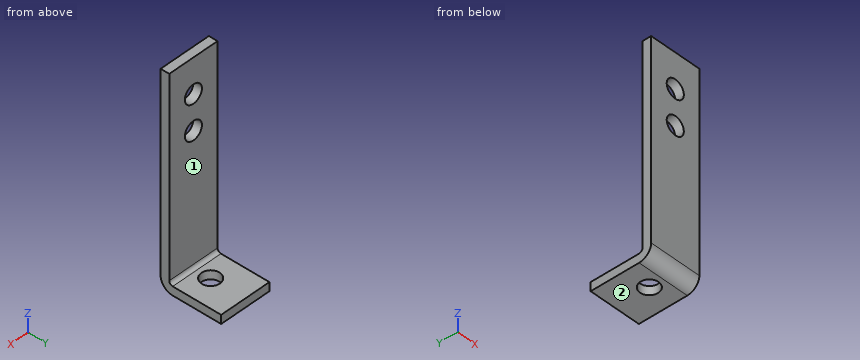
Autodesk Inventor part; units mm, degrees
ref_plane "YZ Plane" through (0, 0, 0) normal (1, 0, 0) x (0, 1, 0)
ref_plane "XZ Plane" through (0, 0, 0) normal (0, 1, 0) x (-1, 0, 0)
ref_plane "XY Plane" through (0, 0, 0) normal (0, 0, 1) x (1, 0, 0)
sketch "Sketch1" plane through (0, 0, 0) normal (0, 0, 1) x (1, 0, 0)
  line L0 (0, 0) -> (0, -22.225)
  line L1 (0, 0) -> (-19.05, 0)
  line L2 (-19.05, 0) -> (-19.05, -22.225)
  line L3 (-19.05, -22.225) -> (0, -22.225)
  dimension "d0" = 22.225
  dimension "d1" = 19.05
extrude "Plate1" add sketch "Sketch1" along normal blind 3.175
sketch "Sketch2" plane through (0, -19.05, 0) normal (0, -1, 0) x (1, 0, 0)
  line L0 (-19.05, 0) -> (0, 0)
  line L1 (0, 0) -> (0, 76.2)
  line L2 (0, 76.2) -> (-19.05, 76.2)
  line L3 (-19.05, 76.2) -> (-19.05, 0)
edge flange "Flange1" height 76.2 angle 90 thickness 3.175 bend radius 1.27 thickness toward (0, -1, 0) relief straight relief width 3.175 relief depth 1.5875 edges at (-9.525, -22.225, 3.175) wall of the first edge with corners at (-19.05, -19.05, 0) (0, -19.05, 0) (0, -19.05, 76.2) (-19.05, -19.05, 76.2)
bend "Bend1"
corner "Corner1"
sketch "Sketch3" plane through (0, 0, 3.175) normal (0, 0, 1) x (1, 0, 0)
  circle A0 centre (90.7515, -113.3098) radius 3.3782
  circle A1 centre (90.7515, -113.3098) radius 3.3782
  circle A2 centre (-9.525, -12.7) radius 3.3782
extrude "Cut1" cut sketch "Sketch3" against normal blind 3.175 contours A2
sketch "Sketch4" plane through (-19.05, -19.05, 76.2) normal (0, 1, 0) x (1, 0, 0)
  line L0 (0, 0) -> (19.05, 0)
  line L1 (19.05, 0) -> (19.05, 71.755)
  line L2 (9.525, 0) -> (9.525, 12.7)
  circle A0 centre (9.525, 12.7) radius 3.3782
  line L3 (9.525, 12.7) -> (9.525, 25.4)
  circle A1 centre (9.525, 25.4) radius 3.3782
  point P0 (19.05, 76.2)
  dimension "d15" = 12.7
  dimension "d16" = 6.7564
  dimension "d17" = 12.7
  dimension "d18" = 6.7564
extrude "Cut2" cut sketch "Sketch4" against normal blind 3.175
equation "\"d13\" = Thickness"
equation "\"d19\" = Thickness"
equation "\"d3\" = BendReliefWidth"
equation "\"d4\" = BendReliefDepth"
equation "\"d5\" = MinimumRemnant"
equation "\"d6\" = BendRadius"
equation "\"d10\" = CornerReliefSize"
equation "\"d11\" = GapSize"
equation "\"d12\" = JacobiRadiusSize"
equation "\"BendRadius\" = Thickness"
equation "\"BendReliefWidth\" = Thickness"
equation "\"BendReliefDepth\" = 0.5 * Thickness"
equation "\"CornerReliefSize\" = 4 * Thickness"
equation "\"MinimumRemnant\" = 2 * Thickness"
equation "\"TransitionRadius\" = BendRadius"
equation "\"JacobiRadiusSize\" = Thickness"
equation "\"GapSize\" = Thickness"
equation "\"d2\" = BendRadius"
properties part number "pawl mount reinforcement"
Could you check a few things on this model? Use its own coordinates, in mm. Face numbers are marked on the shaded views. A direction names the side the tool comes from. Coordinates: 2 decimals unless noted, no trailing zeros. Order: outer loops, then holes, each group sorted by start corner. A loop starts at its lowest first (then second) coordinate and runs counter-clockwise, first axis right, second up. Notation, with made-up numbers: (28, -38) - (58, -38) arc R15 cw to (58, -19) - close; hole circle Ø4 at (-26, 53). An arc over 180 degrees is marked (long way). Answer in a Markdown table with one row per item. Add a question column.
(1) If we section it at B-B, the plane z = 63.5: Please give me the cut outline in (x, y) (3 decimals).
(2) If we section it at A-A, the plane y = -12.7: Please give me the cut outline in (x, z) (3 decimals), then the cut area to 3 significant figures.
(3) I need wall thicknesses on L1, parallel to X at y = -20.3, z = 63.5; L2, parallel to Z at x = -13.5, y = -8 (3 decimals); L3, parallel to Y at x = -16, z = 56 (3 decimals). Which ranges of each line are inside material? Lowest first, please.
(4) Will these pins go through, and if not, where does the flat tip stop? pin 1 (10 mm diameter, centred on x = -10, y = -18, fed in from +Z); pin 2 (6 mm diameter, centred on x = -10, y = -7, fed in from +Z) (3 decimals); pin 3 (5.5 mm diameter, centred on x = -9, z = 48.5, fed in from +Y).
(5) If we section it at C-C, the plane x = -9.5: Please give me the cut outline in (y, z) (3 decimals), then the cut area to 3 significant figures.
(6) On a 3-axis mill with a long thin cutter (end or side, diameter ignored), from which of +Z, -Z, +X, -X, +Y, -Y can I reach the whole of each face in a straight line? I mean the marked faces 1 and 2. Say none if no direction works.
(7) If we section it at D-D, the plane x = -1.5: Please give me the cut outline in (y, z) (3 decimals), then the cut area to 3 significant figures.
Results are:
| question | item | result |
|---|---|---|
| 1 | outline | (-19.05, -22.225) - (-12.903, -22.225) - (-12.903, -19.05) - (-19.05, -19.05) - close; (-6.147, -22.225) - (0, -22.225) - (0, -19.05) - (-6.147, -19.05) - close |
| 2 | outline | (-19.05, 0) - (-12.903, 0) - (-12.903, 3.175) - (-19.05, 3.175) - close; (-6.147, 0) - (0, 0) - (0, 3.175) - (-6.147, 3.175) - close |
| 2 | area | 39.0 mm2 |
| 3 | L1 | x = -19.05 to -12.9, -6.15 to 0 |
| 3 | L2 | z = 0 to 3.175 |
| 3 | L3 | y = -22.225 to -19.05 |
| 4 | pin 1 | stops at z = 76.2 |
| 4 | pin 2 | stops at z = 3.175 |
| 4 | pin 3 | stops at y = -19.05 |
| 5 | outline | (-22.225, 4.445) arc R4.445 ccw to (-17.78, 0) - (-16.078, 0) - (-16.078, 3.175) - (-17.78, 3.175) arc R1.27 cw to (-19.05, 4.445) - (-19.05, 47.422) - (-22.225, 47.422) - close; (-22.225, 54.178) - (-19.05, 54.178) - (-19.05, 60.122) - (-22.225, 60.122) - close; (-22.225, 66.878) - (-19.05, 66.878) - (-19.05, 76.2) - (-22.225, 76.2) - close; (-9.322, 0) - (0, 0) - (0, 3.175) - (-9.322, 3.175) - close |
| 5 | area | 234 mm2 |
| 6 | face 1 | +Z, +X, -X, +Y |
| 6 | face 2 | -Z, +X, -X, +Y, -Y |
| 7 | outline | (-22.225, 4.445) arc R4.445 ccw to (-17.78, 0) - (0, 0) - (0, 3.175) - (-17.78, 3.175) arc R1.27 cw to (-19.05, 4.445) - (-19.05, 76.2) - (-22.225, 76.2) - close |
| 7 | area | 299 mm2 |
